Here's the drawing with two shaded views (mm, measured from the low corner). I have some questions. A direction names the side the tool comes from. Round coordinates to 2 decimals unless told otherwise and drop trailing zeros. Loops run counter-clockwise (first coordinate to the right, second up) from the corner with the lowest first, then second, coordinate; pieces in that order, holes last. Notation, with made-up numbers: (-35.75, 66) -> (-24.75, 66) arc R25 ccw to (-24.75, 90) -> close; hole circle Ø7 at (19, -13.5). An arc over 180 degrees is marked (long way). Use a Markdown table: item, result.
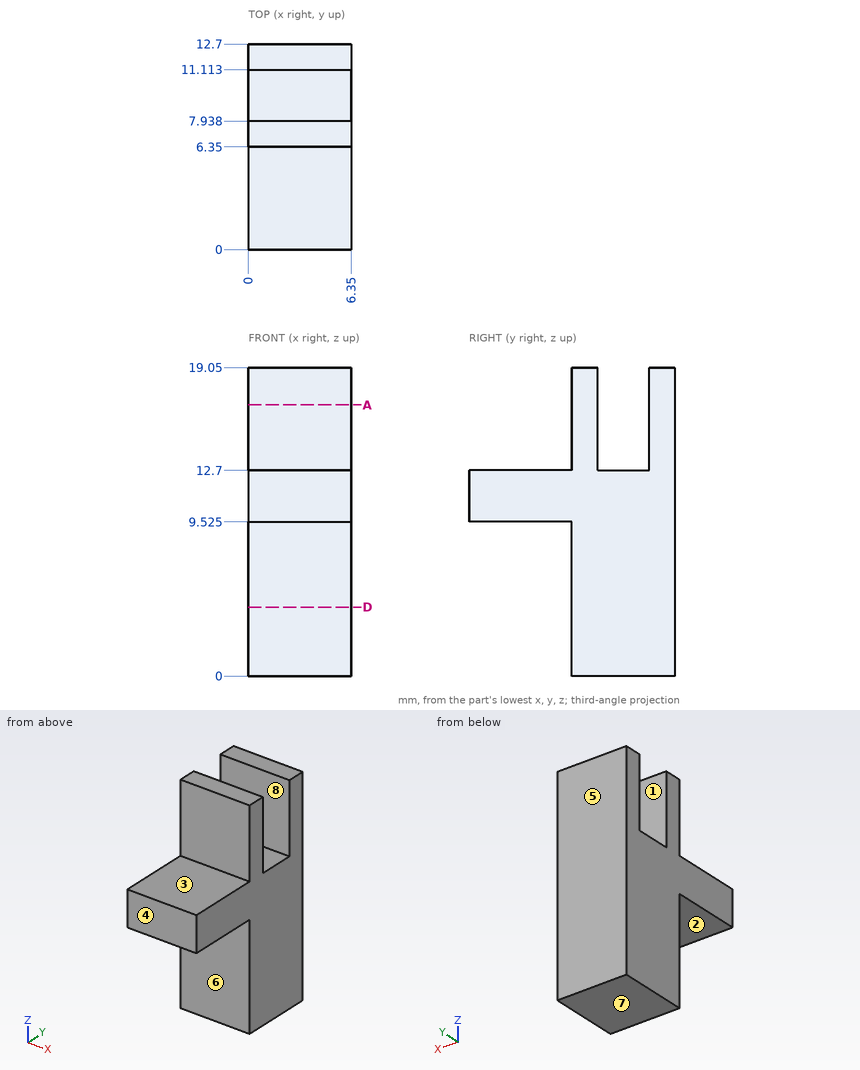
1. If we mould it in two halves opening along Y, with no side actions, what happens to the marked faces 5, 6, 7 and 8? For each: +Y half, -Y half, draft (parallel to the pull), parting line (faces both ways), or undercut.
Answer sheet:
| item | result |
|---|---|
| face 5 | +Y half |
| face 6 | -Y half |
| face 7 | draft |
| face 8 | undercut |
2. I need wall thicknesses on line 1 (Y direction, x = 3, z = 14.5); line 2 (Y direction, x = 3, z = 2); line 3 (Z direction, x = 2.75, y = 8.75). Which ranges of each line are inside material? Lowest first, please.
Answer sheet:
| item | result |
|---|---|
| line 1 | y = 6.35 to 7.94, 11.11 to 12.7 |
| line 2 | y = 6.35 to 12.7 |
| line 3 | z = 0 to 12.7 |
3. I want a section at A-A (z = 16.75). Please give me the cut outline in (x, y).
Answer sheet:
| item | result |
|---|---|
| outline | (0, 6.35) -> (6.35, 6.35) -> (6.35, 7.94) -> (0, 7.94) -> close; (0, 11.11) -> (6.35, 11.11) -> (6.35, 12.7) -> (0, 12.7) -> close |
4. Which directions (+Z, -Z, +X, -X, +Y, -Y) give clear straight access to the entire face, cutting with the end or side of a thin tool? Please do the marked faces 1, 2, 3 and 4.
Answer sheet:
| item | result |
|---|---|
| face 1 | +Z, +X, -X |
| face 2 | -Z, +X, -X, -Y |
| face 3 | +Z, +X, -X, -Y |
| face 4 | +Z, -Z, +X, -X, -Y |
5. I want a section at D-D (z = 4.25). Please give me the cut outline in (x, y).
Answer sheet:
| item | result |
|---|---|
| outline | (0, 6.35) -> (6.35, 6.35) -> (6.35, 12.7) -> (0, 12.7) -> close |
6. Will these pins go through, and if not, where does the flat tip stop? pin 1 Ø1.5 at (x, z) = (2, 5) entering from -Y; pin 2 Ø1.9 at (x, y) = (4.5, 3.5) entering from +Z.
Answer sheet:
| item | result |
|---|---|
| pin 1 | stops at y = 6.35 |
| pin 2 | stops at z = 12.7 |
